```python
from build123d import *

# Parameters (mm, degrees)
CROQUIS1_R              = 9.25
CROQUIS1_R_2            = 3
CROQUIS1_W              = 1.5
CROQUIS1_H              = 5.80947502
SALIENTE_EXTRUIR1_DEPTH = 2.5
CROQUIS1_4_W            = 1.5
CROQUIS1_4_H            = 5.80947502
SALIENTE_EXTRUIR2_DEPTH = 5
CROQUIS1_5_R            = 9.25
CROQUIS1_5_R_2          = 3
SALIENTE_EXTRUIR3_DEPTH = 1
CORTAR_EXTRUIR1_REACH   = 16.511
CROQUIS2_R              = 1.25


with BuildPart() as part:
    # Croquis1 → Saliente-Extruir1 (new body)
    # profile 1 of 6: a face of its own
    with BuildSketch(Plane.XY):
        Circle(CROQUIS1_R)
        Circle(CROQUIS1_R_2, mode=Mode.SUBTRACT)
    # profile 2 of 6: a face of its own
    with BuildSketch(Plane.XY):
        with BuildLine():
            Line((-0.75, -2.90473751), (-0.75, 2.90473751))
            ThreePointArc((-0.75, 2.90473751), (-3, 0), (-0.75, -2.90473751))
        make_face()
    # profile 3 of 6: a face of its own
    with BuildSketch(Plane.XY):
        with BuildLine():
            ThreePointArc((3, 0), (2.371708245, 1.837117307), (0.75, 2.90473751))
            Line((0.75, 2.90473751), (0.75, -2.90473751))
            ThreePointArc((0.75, -2.90473751), (2.371708245, -1.837117307), (3, 0))
        make_face()
    # profile 4 of 6: a face of its own
    with BuildSketch(Plane.XY):
        Rectangle(CROQUIS1_W, CROQUIS1_H)
    # profile 5 of 6: a face of its own
    with BuildSketch(Plane.XY):
        with BuildLine():
            Line((0.75, -2.90473751), (-0.75, -2.90473751))
            ThreePointArc((-0.75, -2.90473751), (0, -3), (0.75, -2.90473751))
        make_face()
    # profile 6 of 6: a face of its own
    with BuildSketch(Plane.XY):
        with BuildLine():
            ThreePointArc((0.75, 2.90473751), (0, 3), (-0.75, 2.90473751))
            Line((-0.75, 2.90473751), (0.75, 2.90473751))
        make_face()
    extrude(amount=SALIENTE_EXTRUIR1_DEPTH)

    # Croquis1<4> → Saliente-Extruir2 (add)
    with BuildSketch(Plane.XY):
        Rectangle(CROQUIS1_4_W, CROQUIS1_4_H)
        with BuildLine():
            ThreePointArc((0.75, 2.90473751), (0, 3), (-0.75, 2.90473751))
            Line((-0.75, 2.90473751), (0.75, 2.90473751))
        make_face()
        with BuildLine():
            Line((0.75, -2.90473751), (-0.75, -2.90473751))
            ThreePointArc((-0.75, -2.90473751), (0, -3), (0.75, -2.90473751))
        make_face()
    extrude(amount=-SALIENTE_EXTRUIR2_DEPTH)

    # Croquis1<5> → Saliente-Extruir3 (add)
    with BuildSketch(Plane.XY):
        Circle(CROQUIS1_5_R)
        Circle(CROQUIS1_5_R_2, mode=Mode.SUBTRACT)
    extrude(amount=-SALIENTE_EXTRUIR3_DEPTH)

    # Croquis2 → Cortar-Extruir1 (cut, up to next)
    with BuildSketch(Plane(origin=(0.75, 0, 0), x_dir=(0, 0, -1), z_dir=(1, 0, 0)), mode=Mode.PRIVATE) as cortar_extruir1_sk1:
        with Locations((3.1, 0)):
            Circle(CROQUIS2_R)
    cortar_extruir1_tool1 = extrude(cortar_extruir1_sk1.sketch, amount=-CORTAR_EXTRUIR1_REACH, mode=Mode.PRIVATE) & part.part
    add(cortar_extruir1_tool1.solids().sort_by_distance((0.75, 0, -3.1))[0], mode=Mode.SUBTRACT)


solid = part.part
```
Work out the finished part from the listing and answer in its coordinate system (mm). A direction names the side the tool comes from. Coordinates: 2 decimals unless noted, no trailing zeros. Order: outer loops, then holes, each group sorted by start corner. A loop starts at its lowest first (then second) coordinate and runs counter-clockwise, first axis right, second up. Notation, with made-up numbers: (-20.75, -8) - (-12.75, -8) arc R11 ccw to (-12.75, 3) - close; hole circle Ø6 at (-24.5, 60.5). An arc over 180 degrees is marked (long way). Answer as a JSON object with one key per item and string values.
1. Find section B-B on x = 0. Determine the outline of the cut face in (y, z), plus the area to 3 significant figures.
Output values:
{"outline": "(-9.25, -1) - (-3, -1) - (-3, -5) - (3, -5) - (3, -1) - (9.25, -1) - (9.25, 2.5) - (-9.25, 2.5) - close; hole circle Ø2.5 at (0, -3.1)", "area": "83.8 mm²"}
2. The mould has two halves that part along Y. Classify faces 4 (the face through (0, 3, -3)), 5 (the face through (-0.75, -1, -2)), 6 (the face through (-2.01, -9.03, 0.77)): +Y half, -Y half, draft (parallel to the pull), parting line (faces both ways), or undercut.
Output values:
{"face 4": "+Y half", "face 5": "undercut", "face 6": "parting line"}
3. Find section D-D on z = 2.25. Determine the outline of the cut face in (x, y).
Output values:
{"outline": "circle Ø18.5 at (0, 0)"}
4. A tool of negligible diameter and unlimited length cuts with its end or side. For faces 1 (the face through (0, 0, -5)), 2 (the face through (0, -3, -3)), 3 (the face through (-2, 0, 0)), from which of +Z, -Z, +X, -X, +Y, -Y can it reach the whole face along a straight path? Write none if from no direction.
Output values:
{"face 1": "-Z, +X, -X, +Y, -Y", "face 2": "-Z, -Y", "face 3": "-Z"}
5. Find section C-C on z = -3.1. Determine the outline of the cut face in (x, y), plus the area to 3 significant figures.
Output values:
{"outline": "(-0.75, -2.9) arc R3 ccw to (0.75, -2.9) - (0.75, -1.25) - (-0.75, -1.25) - close; (-0.75, 1.25) - (0.75, 1.25) - (0.75, 2.9) arc R3 ccw to (-0.75, 2.9) - close", "area": "5.16 mm²"}
6. Each of these flat-tipped pins is pushed along its axis until it touches: P1, Ø1.5, axis at y = 1, z = -3, coming from the -X side; P2, Ø9, axis at x = 3.5, y = -1.5, coming from the -Z side; P3, Ø0.7, axis at x = -1.5, y = 0, coming from the -Z side; P4, Ø4, axis at x = 6, z = 0, coming from the +Y side. Where does it stop, or does it pass through?
Output values:
{"P1": "stops at x = -0.75", "P2": "stops at z = -5", "P3": "stops at z = 0", "P4": "stops at y = 8.34"}
7. Consider line 1 (X direction, y = -2.5, z = -0.5); line 2 (Z direction, x = 7.75, y = -4.5); line 3 (X direction, y = 2.5, z = -2.75). Determine where each line is inside the solid, lowest interval first.
Output values:
{"line 1": "x = -8.91 to -1.66, -0.75 to 0.75, 1.66 to 8.91", "line 2": "z = -1 to 2.5", "line 3": "x = -0.75 to 0.75"}
8. Find section A-A on y = 0. Determine the outline of the cut face in (x, z).
Output values:
{"outline": "(-9.25, -1) - (-3, -1) - (-3, 0) - (-0.75, 0) - (-0.75, -1.85) - (0.75, -1.85) - (0.75, 0) - (3, 0) - (3, -1) - (9.25, -1) - (9.25, 2.5) - (-9.25, 2.5) - close; (-0.75, -5) - (0.75, -5) - (0.75, -4.35) - (-0.75, -4.35) - close"}
